Check sheet for the modelled part. Datum: model origin and axes. Units: mm. Face numbers are marked on the shaded views. A direction names the side the tool comes from. Give positions to 0.01 mm unless a question says otherwise; leave off trailing zeros. Loops run counter-clockwise (first coordinate to the right, second up) from the corner with the lowest first, then second, coordinate; pieces in that order, holes last. Notation, with made-up numbers: (85, -12) -> (124, -12) arc R37 cw to (124, 26) -> close; hole circle Ø10 at (31.25, 60). An arc over 180 degrees is marked (long way). Answer as CSV lines item,"result". Start each with the question number.
(1) Gauge pin test, flat ends, axial feed: pin 1 Ø1.5 at (x, z) = (2.5, 19.5) entering from +Y; pin 2 Ø23 at (x, y) = (6.5, 1.5) entering from +Z; pin 3 Ø12 at (x, z) = (-6.5, 20) entering from -Y. Record the tip position at first contact, or that the pin passes through.
(2) Section check A-A on y = 0. Enter the section's corners in (x, z), plus the area to 3 significant figures.
(3) Material ranges on line 1 (Y direction, x = 0, z = 1.35); line 2 (Y direction, x = 5, z = 2.75); line 3 (Z direction, x = 21, y = 6), recorded low to high. Write a range as from..to.
(4) Section check C-C on z = 2.75. Enter the section's corners in (x, y), plus the area to 3 significant figures.
(5) Access from +Z, -Z, +X, -X, +Y, -Y to the whole of each face (thin tool, end or side, straight path). Record for the marked faces 1, 2 and 3.
(6) Release check for a two-part mould opening along X. For the marked faces 4, 5 and 6 record: pulls with the +X half, pulls with the -X half, needs draft (parallel to the pull), parting line crosses it, or undercut.
(7) Section check D-D on z = 7.25. Enter the section's corners in (x, y).
(8) Section check B-B on x = 0. Enter the section's corners in (y, z).
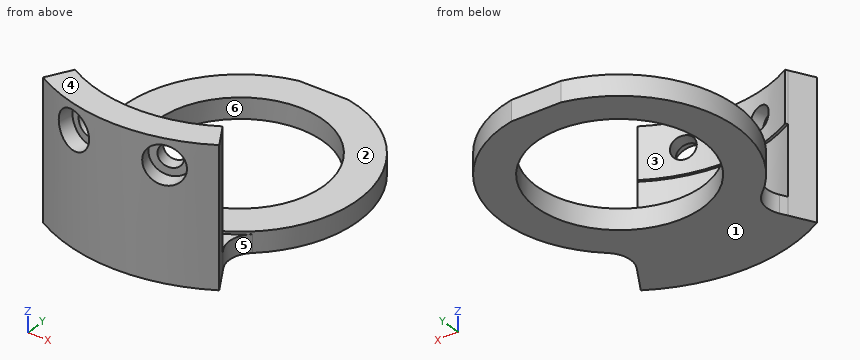
from build123d import *

# Parameters (mm, degrees)
SKETCH_1_R                          = 23
SKETCH_1_R_2                        = 16.25
EXTRUDE_1_DEPTH                     = 4
SKETCH_2_W                          = 9.539392014
SKETCH_2_H                          = 6.996470021
CUT_EXTRUDE_1_DEPTH                 = 14
EXTRUDE_2_DEPTH                     = 3.5
EXTRUDE_3_DEPTH                     = 27
FILLET_1_R                          = 5
EXTRUDE_START                       = -10
EXTRUDE_4_DEPTH                     = 10
HOLE_WIZARD_1_D                     = 4.5
HOLE_WIZARD_1_CBORE_D               = 7.5
HOLE_WIZARD_1_CBORE_DEPTH           = 3
HOLE_WIZARD_1_ON_FACE_2_D           = 4.5
HOLE_WIZARD_1_ON_FACE_2_CBORE_D     = 7.5
HOLE_WIZARD_1_ON_FACE_2_CBORE_DEPTH = 3


with BuildPart() as part:
    # Sketch 1 → Extrude 1 (new body)
    with BuildSketch(Plane.XY):
        Circle(SKETCH_1_R)
        Circle(SKETCH_1_R_2, mode=Mode.SUBTRACT)
    extrude(amount=EXTRUDE_1_DEPTH)

    # Sketch 2 → Cut-Extrude 1 (cut)
    with BuildSketch(Plane.XY):
        with Locations((0, 25.998235011)):
            Rectangle(SKETCH_2_W, SKETCH_2_H)
    extrude(amount=CUT_EXTRUDE_1_DEPTH, mode=Mode.SUBTRACT)

    # Sketch 3 → Extrude 2 (add)
    with BuildSketch(Plane.XY):
        with BuildLine():
            ThreePointArc((11.5, -19.918584287), (5.952838037, -22.216294005), (0, -23))
            Line((0, -23), (0, -29))
            ThreePointArc((0, -29), (7.505752308, -28.011848962), (14.5, -25.11473671))
            Line((14.5, -25.11473671), (11.5, -19.918584287))
        make_face()
        with BuildLine():
            ThreePointArc((0, -23), (-5.952838037, -22.216294005), (-11.5, -19.918584287))
            Line((-11.5, -19.918584287), (-14.5, -25.11473671))
            ThreePointArc((-14.5, -25.11473671), (-7.505752308, -28.011848962), (0, -29))
            Line((0, -29), (0, -23))
        make_face()
    extrude(amount=EXTRUDE_2_DEPTH)

    # Sketch 3_3 → Extrude 3 (add)
    with BuildSketch(Plane.XY):
        with BuildLine():
            ThreePointArc((14.5, -25.11473671), (0, -29), (-14.5, -25.11473671))
            Line((-14.5, -25.11473671), (-17, -29.444863729))
            ThreePointArc((-17, -29.444863729), (0, -34), (17, -29.444863729))
            Line((17, -29.444863729), (14.5, -25.11473671))
        make_face()
    extrude(amount=EXTRUDE_3_DEPTH)

    # Fillet 1
    fillet_1_edges = [part.edges().sort_by_distance(p)[0] for p in [
        (11.5, -19.918584287, 1.75),
        (-11.5, -19.918584287, 1.75),
    ]]
    fillet(fillet_1_edges, radius=FILLET_1_R)

    # Sketch 4 → Extrude 4 (add)
    with BuildSketch(Plane.XY.offset(27).offset(EXTRUDE_START)):
        with BuildLine():
            Line((17, -29.444863729), (14.5, -25.11473671))
            ThreePointArc((14.5, -25.11473671), (0, -29), (-14.5, -25.11473671))
            Line((-14.5, -25.11473671), (-17, -29.444863729))
            ThreePointArc((-17, -29.444863729), (0, -34), (17, -29.444863729))
        make_face()
        with BuildLine():
            Line((-14.25, -24.681724008), (-14.5, -25.11473671))
            ThreePointArc((-14.5, -25.11473671), (0, -29), (14.5, -25.11473671))
            Line((14.5, -25.11473671), (14.25, -24.681724008))
            ThreePointArc((14.25, -24.681724008), (0, -28.5), (-14.25, -24.681724008))
        make_face()
    extrude(amount=EXTRUDE_4_DEPTH)

    # Hole Wizard 1 (through all)
    with Locations(Plane(origin=(-8.799847533, -32.841478094, 22), x_dir=(-0.965925826289, 0.258819045103, 0), z_dir=(-0.258819045103, -0.965925826289, 0))):
        with Locations((1e-09, 0)):
            CounterBoreHole(HOLE_WIZARD_1_D / 2, HOLE_WIZARD_1_CBORE_D / 2, HOLE_WIZARD_1_CBORE_DEPTH)

    # Hole Wizard 1 on face 2 (through all)
    with Locations(Plane(origin=(8.799847533, -32.841478094, 22), x_dir=(-0.965925849201, -0.258818959594, 0), z_dir=(0.258818959594, -0.965925849201, 0))):
        with Locations((-1e-09, 0)):
            CounterBoreHole(HOLE_WIZARD_1_ON_FACE_2_D / 2, HOLE_WIZARD_1_ON_FACE_2_CBORE_D / 2, HOLE_WIZARD_1_ON_FACE_2_CBORE_DEPTH)


solid = part.part
Working result:
1,pin 1,"stops at y = -28.31"
1,pin 2,"stops at z = 4"
1,pin 3,"stops at y = -34"
2,outline,"(-23, 0) -> (-16.25, 0) -> (-16.25, 4) -> (-23, 4) -> close; (16.25, 0) -> (23, 0) -> (23, 4) -> (16.25, 4) -> close"
2,area,"54.0 mm^2"
3,line 1,"y = -34..-16.25, 16.25..22.5"
3,line 2,"y = -33.63..-15.46, 15.46..22.45"
3,line 3,"z = 0..4"
4,outline,"(-17, -29.44) arc R34 ccw to (17, -29.44) -> (13.77, -23.86) arc R5 cw to (14.87, -17.54) arc R23 ccw to (4.77, 22.5) -> (-4.77, 22.5) arc R23 ccw to (-14.87, -17.54) arc R5 cw to (-13.77, -23.86) -> close; hole circle Ø32.5 at (0, 0)"
4,area,"1,170 mm^2"
5,face 1,"-Z, +X, -X, +Y, -Y"
5,face 2,"+Z, +X, -X, +Y"
5,face 3,"+Z, +Y"
6,face 4,"needs draft"
6,face 5,"pulls with the +X half"
6,face 6,"undercut"
7,outline,"(-17, -29.44) arc R34 ccw to (17, -29.44) -> (14.5, -25.11) arc R29 cw to (-14.5, -25.11) -> close"
8,outline,"(-34, 0) -> (-16.25, 0) -> (-16.25, 4) -> (-23, 4) -> (-23, 3.5) -> (-29, 3.5) -> (-29, 17) -> (-28.5, 17) -> (-28.5, 27) -> (-34, 27) -> close; (16.25, 0) -> (22.5, 0) -> (22.5, 4) -> (16.25, 4) -> close"
